from build123d import *

# Parameters (mm, degrees)
CROQUIS1_R                    = 5
SALIENTE_EXTRUIR1_DEPTH       = 10
CROQUIS4_W                    = 15
CROQUIS4_H                    = 25
SALIENTE_EXTRUIR3_DEPTH       = 15
SALIENTE_EXTRUIR9_DEPTH       = 25
SALIENTE_EXTRUIR10_DEPTH      = 7.75
SALIENTE_EXTRUIR10_DEPTH_BACK = 17.5
ESCALA1_SCALE                 = 0.75


with BuildPart() as part:
    # Croquis1 → Saliente-Extruir1 (new body)
    with BuildSketch(Plane.XY):
        with BuildLine():
            Line((0, 7.5), (30, 7.5))
            Line((30, 7.5), (37.5, 7.5))
            Line((37.5, 7.5), (37.5, -7.5))
            Line((37.5, -7.5), (30, -7.5))
            Line((30, -7.5), (0, -7.5))
            ThreePointArc((0, -7.5), (-7.5, 0), (0, 7.5))
        make_face()
        Circle(CROQUIS1_R, mode=Mode.SUBTRACT)
    extrude(amount=SALIENTE_EXTRUIR1_DEPTH)

    # Croquis4 → Saliente-Extruir3 (add)
    with BuildSketch(Plane.XZ.offset(7.5)):
        with Locations((32.819126762, 4.89)):
            Rectangle(CROQUIS4_W, CROQUIS4_H)
    extrude(amount=-SALIENTE_EXTRUIR3_DEPTH)

    # Croquis11 → Saliente-Extruir9 (add)
    with BuildSketch(Plane(origin=(0, 0, -7.61), x_dir=(-1, 0, 0), z_dir=(0, 0, -1))):
        Polygon((-40.319126762, 7.5), (-58.184981349, 25.365854587), (-40.319126762, -7.5), align=None)
    extrude(amount=-SALIENTE_EXTRUIR9_DEPTH)

    # Croquis14 → Saliente-Extruir10 (add, two sides: drawn at the far end of the back side and taken through both)
    with BuildSketch(Plane(origin=(0, 0, 0), x_dir=(-1, 0, 0), z_dir=(0, 0, -1)).offset(-SALIENTE_EXTRUIR10_DEPTH_BACK)):
        Polygon((-25.319126762, 7.5), (-7.641457232, 25.17766953), (-25.319126762, -7.5), align=None)
    extrude(amount=SALIENTE_EXTRUIR10_DEPTH + SALIENTE_EXTRUIR10_DEPTH_BACK)


with BuildPart() as part_1:
    # Escala1: scaled about (27.940941058, 3.516863711, 4.909948999)
    add(part.part.scale(ESCALA1_SCALE).moved(Location((6.985235264, 0.879215928, 1.22748725))))


solid = part_1.part
Could you check a few things on this model? Use its own coordinates, in mm. A direction names the side the tool comes from. Coordinates: 2 decimals unless noted, no trailing zeros. Order: outer loops, then holes, each group sorted by start corner. A loop starts at its lowest first (then second) coordinate and runs counter-clockwise, first axis right, second up. Notation, with made-up numbers: (18.5, 33) -> (27.5, 33) arc R19 ccw to (27.5, 40) -> close; hole circle Ø2 at (49, 7.5). An arc over 180 degrees is marked (long way). One line per question, with ' | ' between items.
Q1. Imagine slicing it at A-A on y = 9. Please give me the cut outline in (x, z), and give its area (3 significant figures).
Return value:
outline: (18.54, -4.59) -> (23.48, -4.59) -> (23.48, 14.35) -> (18.54, 14.35) -> close; (39.72, -4.48) -> (44.7, -4.48) -> (44.7, 14.27) -> (39.72, 14.27) -> close | area: 187 mm²
Q2. I'm going to push flat-ended pins straight in: P1, Ø3, axis at y = 5.5, z = 8.5, coming from the -X side; P2, Ø1.5, axis at x = 21.5, z = 7.5, coming from the +Y side; P3, Ø6, axis at x = 16.5, z = 3.5, coming from the +Y side; P4, Ø9, axis at x = 19.5, y = -2, coming from the +Z side. Where does each tip first touch, or does it pass through?
Return value:
P1: x = 2.31 | P2: y = 11.73 | P3: y = 18.98 | P4: z = 14.35
Q3. Imagine slicing it at D-D on y = -2.25. Please give me the cut outline in (x, z), and give its area (3 significant figures).
Return value:
outline: (2.31, 1.23) -> (4.92, 1.23) -> (4.92, 8.73) -> (2.31, 8.73) -> close; (9.05, 1.23) -> (24.62, 1.23) -> (24.62, -4.59) -> (25.97, -4.59) -> (25.97, -4.48) -> (38.58, -4.48) -> (38.58, 14.27) -> (25.97, 14.27) -> (25.97, 14.35) -> (24.62, 14.35) -> (24.62, 8.73) -> (9.05, 8.73) -> close | area: 398 mm²
Q4. Thinking about a two-plate mould opening in Y: for faces 5 (the face through (13, 6.504, 5)), 6 (the face through (25, -4.746, 5)), 7 (the face through (8.716, -2.448, 4.925)), 8 (the face through (35, 2, 14.27)), which applies, pulls with the +Y half, pulls with the -Y half, needs draft (parallel to the pull), parting line crosses it, or undercut?
Return value:
face 5: undercut | face 6: pulls with the -Y half | face 7: undercut | face 8: needs draft
Q5. Imagine slicing it at B-B on x = 16. Please give me the cut outline in (y, z).
Return value:
outline: (-4.75, 1.23) -> (6.5, 1.23) -> (6.5, 8.73) -> (-4.75, 8.73) -> close; (13.69, -4.59) -> (16.48, -4.59) -> (16.48, 14.35) -> (13.69, 14.35) -> close
Q6. If I drill on L1, parallel to Z at x = 39, y = 3.25; L2, parallel to X at y = 13.25, z = 3.75; L3, parallel to Z at x = 22.5, y = -3.5, over which ranges is the centre line in solid material (lowest first)?
Return value:
L1: -4.48 to 14.27 | L2: 16.24 to 19.23, 43.97 to 47.01 | L3: 1.23 to 8.73
Q7. Imagine slicing it at C-C on z = 8.25. Please give me the cut outline in (x, y) (3 decimals), and give its area (3 significant figures).
Return value:
outline: (6.985, -4.746) -> (37.225, -4.746) -> (50.624, 19.904) -> (37.225, 6.504) -> (25.975, 6.504) -> (12.716, 19.762) -> (19.889, 6.504) -> (6.985, 6.504) arc R5.625 ccw to start; hole circle Ø7.5 at (6.985, 0.879) | area: 461 mm²
Q8. On a 3-axis mill with a long thin cutter (end or side, diameter ignored), from which of +Z, -Z, +X, -X, +Y, -Y can I reach the whole of each face in a straight line? I mean faces 1 (the face through (43.83, 13.11, 4.76)), 2 (the face through (35, 2, -4.48)), 3 (the face through (14, 1, 8.727)), 4 (the face through (14, 1, 1.227)). Say none if no direction works.
Return value:
face 1: +Z, -Z, +Y | face 2: -Z, +X, +Y, -Y | face 3: +Z, -X, -Y | face 4: -Z, -X, -Y
